Autodesk Inventor part; units mm, degrees
ref_plane "YZ Plane" through (0, 0, 0) normal (1, 0, 0) x (0, 1, 0)
ref_plane "XZ Plane" through (0, 0, 0) normal (0, 1, 0) x (-1, 0, 0)
ref_plane "XY Plane" through (0, 0, 0) normal (0, 0, 1) x (1, 0, 0)
sketch "Sketch1" plane through (0, 0, 0) normal (0, 1, 0) x (-1, 0, 0)
  line L0 (0, 0) -> (5, 0)
  line L1 (5, 0) -> (5, -115)
  line L2 (5, -115) -> (0, -115)
  line L3 (0, -115) -> (0, 0)
  line L4 (5, -115) -> (20, -115)
  line L5 (20, -115) -> (20, -105)
  line L6 (20, -105) -> (5, -105)
  line L7 (5, -105) -> (5, -115)
  line L8 (0, -10) -> (0, 0)
  point P0 (5, -105)
  dimension "d0" = 5
  dimension "d1" = 115
  dimension "d2" = 15
  dimension "d3" = 10
extrude "Extrusion1" add sketch "Sketch1" along normal blind 15
sketch "Sketch6" plane through (0, 0, 0) normal (1, 0, 0) x (0, 0, -1)
  line L0 (105, 0) -> (0, 0)
  line L1 (0, 0) -> (5, 0)
  line L2 (5, 0) -> (5, 15)
  line L3 (5, 15) -> (0, 15)
  line L4 (0, 15) -> (0, 0)
  dimension "d24" = 5
  dimension "d25" = 15
extrude "Extrusion4" add sketch "Sketch6" along normal blind 77.5
sketch "Sketch7" plane through (0, 0, 0) normal (0, -1, 0) x (1, 0, 0)
  line L0 (-20, -105) -> (-5, -105)
  line L1 (-20, -115) -> (-20, -105)
  line L2 (0, -115) -> (-20, -115)
  line L3 (0, -5) -> (0, -115)
  line L4 (0, -5) -> (77.5, -5)
  line L5 (77.5, 0) -> (77.5, -5)
  line L6 (-5, 0) -> (77.5, 0)
  line L7 (-5, -105) -> (-5, 0)
  line L8 (175, -105) -> (160, -105)
  line L9 (175, -115) -> (175, -105)
  line L10 (155, -115) -> (175, -115)
  line L11 (155, -5) -> (155, -115)
  line L12 (155, -5) -> (77.5, -5)
  line L13 (160, 0) -> (77.5, 0)
  line L14 (160, -105) -> (160, 0)
  point P0 (0, 0)
extrude "Extrusion5" add sketch "Sketch7" against normal up to surface (15 mm away) contours L13 L14 L8 L9 L10 L11 L12 L5
sketch "Sketch2" plane through (-20, 0, -105) normal (0, 0, 1) x (1, 0, 0)
  line L0 (0, 0) -> (0, 15)
  circle A0 centre (7.5, 7.5) radius 2.15
  line L1 (7.5, 7.5) -> (0, 7.5) construction
  line L2 (15, 15) -> (180, 15)
  line L3 (97.5, 15) -> (97.5, 37.3705) construction
  circle A1 centre (187.5, 7.5) radius 2.15
  point P0 (20, 0)
  dimension "d8" = 4.3
  dimension "d20" = 7.5
extrude "Extrusion2" cut sketch "Sketch2" against normal blind 15
fillet "Fillet2" radius 5 8 edges at (0, 7.5, -5) (0, 7.5, -115) (155, 7.5, -115) (160, 7.5, 0) (155, 7.5, -5) (-5, 7.5, 0) (-5, 7.5, -105) (160, 7.5, -105)
properties part number "Box_clamp"
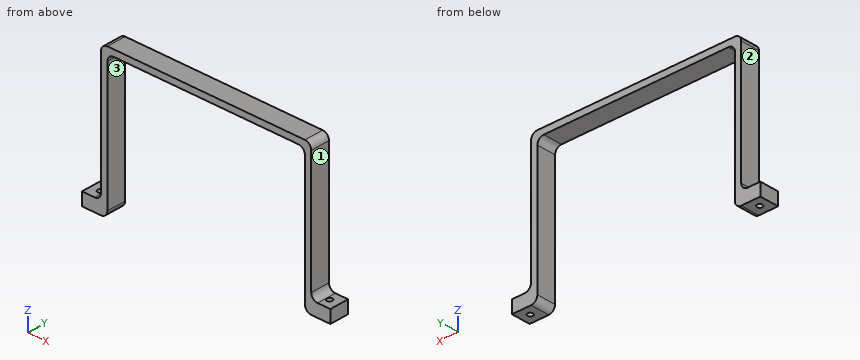
For this review, take the finished solid that the model builds, in its own axes (mm). Face numbers are marked on the shaded views. A direction names the side the tool comes from. Coordinates: 2 decimals unless noted, no trailing zeros. Loops run counter-clockwise (first coordinate to the right, second up) from the corner with the lowest first, then second, coordinate; pieces in that order, holes last. Notation, with made-up numbers: (8.25, 38) - (46.25, 38) arc R23 cw to (46.25, 55) - close; hole circle Ø7 at (47.5, 64). An arc over 180 degrees is marked (long way). Use one line per item in the form item = value. Start each with the question number.
1) To check wall thickness, follow probe 1 along Y at (x, z) = (167.5, -109.75); probe 2 along X at (y, z) = (13.5, -56); probe 3 along Z at (x, y) = (131.5, 1.75). State the ranges of each line that lie inside material, in increasing order. Write a range as from..to.
2) For pin 1 (4.5 mm diameter, centred on y = 7.5, z = -75.5, fed in from +X); pin 2 (3 mm diameter, centred on x = 11, y = 10, fed in from -Z); pin 3 (3 mm diameter, centred on x = -12.5, y = 5.5, fed in from +Z); pin 4 (5.5 mm diameter, centred on x = -12.5, y = 7.5, fed in from -Z), all flat-tipped, find the tip position at first contact; note any pin that passes through.
3) Take a section at A-A (x = 167.5). State the section outline as (y, z) points, plus the area to 3 significant figures.
4) Take a section at D-D (x = 74.5). State the section outline as (y, z) points, plus the area to 3 significant figures.
5) Take a section at B-B (y = 7.5). State the section outline as (x, z) points.
6) For the marked faces 1, 2 and 3, list the 3-axis set-ups (+Z, -Z, +X, -X, +Y, -Y) from which the entire face can be reached by the end or side of a thin tool; tool diameter is ignored.
7) Take a section at C-C (z = -63.5). State the section outline as (x, y) points.
From the geometry:
q1.probe_1 = 0..5.35, 9.65..15
q1.probe_2 = -5..0, 155..160
q1.probe_3 = -5..0
q2.pin_1 = 160
q2.pin_2 = -5
q2.pin_3 = -105
q2.pin_4 = -115
q3.outline = (0, -115) - (5.35, -115) - (5.35, -105) - (0, -105) - close; (9.65, -115) - (15, -115) - (15, -105) - (9.65, -105) - close
q3.area = 107 mm2
q4.outline = (0, -5) - (15, -5) - (15, 0) - (0, 0) - close
q4.area = 75.0 mm2
q5.outline = (-20, -115) - (-14.65, -115) - (-14.65, -105) - (-20, -105) - close; (-10.35, -115) - (-5, -115) arc R5 ccw to (0, -110) - (0, -10) arc R5 cw to (5, -5) - (150, -5) arc R5 cw to (155, -10) - (155, -110) arc R5 ccw to (160, -115) - (165.35, -115) - (165.35, -105) - (165, -105) arc R5 cw to (160, -100) - (160, -5) arc R5 ccw to (155, 0) - (0, 0) arc R5 ccw to (-5, -5) - (-5, -100) arc R5 cw to (-10, -105) - (-10.35, -105) - close; (169.65, -115) - (175, -115) - (175, -105) - (169.65, -105) - close
q6.face_1 = +Z, +X, +Y, -Y
q6.face_2 = +Z, -X, +Y, -Y
q6.face_3 = -Z, +Y, -Y
q7.outline = (-5, 0) - (0, 0) - (0, 15) - (-5, 15) - close; (155, 0) - (160, 0) - (160, 15) - (155, 15) - close
